```python
from build123d import *

# Parameters (mm, degrees)
DODANIE_WYCI_GNI_CIE1_DEPTH = 4
SZKIC2_R                    = 4
WYTNIJ_WYCI_GNI_CIE1_DEPTH  = 199.030300712


with BuildPart() as part:
    # Szkic1 → Dodanie-wyciągnięcie1 (new body)
    with BuildSketch(Plane(origin=(0, 0, 0), x_dir=(1, 0, 0), z_dir=(0, 1, 0))):
        with BuildLine():
            Line((-130, -140), (130, -140))
            ThreePointArc((130, -140), (137.071067812, -137.071067812), (140, -130))
            Line((140, -130), (140, 130))
            ThreePointArc((140, 130), (137.071067812, 137.071067812), (130, 140))
            Line((130, 140), (-130, 140))
            ThreePointArc((-130, 140), (-137.071067812, 137.071067812), (-140, 130))
            Line((-140, 130), (-140, -130))
            ThreePointArc((-140, -130), (-137.071067812, -137.071067812), (-130, -140))
        make_face()
    extrude(amount=DODANIE_WYCI_GNI_CIE1_DEPTH)

    # Szkic2 → Wytnij-wyciągnięcie1 (cut, through all)
    with BuildSketch(Plane(origin=(0, 4, 0), x_dir=(1, 0, 0), z_dir=(0, 1, 0))):
        with Locations(Location((120, 120, 0), (0, 0, 270))):
            Circle(SZKIC2_R)
        with Locations(Location((120, -120, 0), (0, 0, 270))):
            Circle(SZKIC2_R)
        with Locations(Location((-120, -120, 0), (0, 0, 270))):
            Circle(SZKIC2_R)
        with Locations(Location((-120, 120, 0), (0, 0, 270))):
            Circle(SZKIC2_R)
    extrude(amount=-WYTNIJ_WYCI_GNI_CIE1_DEPTH, mode=Mode.SUBTRACT)


solid = part.part
```
Work out the finished part from the listing and answer in its coordinate system (mm). Give positions to 0.01 mm unless a question says otherwise; leave off trailing zeros. Loops run counter-clockwise (first coordinate to the right, second up) from the corner with the lowest first, then second, coordinate; pieces in that order, holes last. Notation, with made-up numbers: (24, -37.75) - (35, -37.75) arc R15 cw to (35, -8.75) - close; hole circle Ø2 at (76, -1). An arc over 180 degrees is marked (long way). One line per question, with ' | ' between items.
(1) The mould has two halves that part along Z. Classify faces 1 (the face through (137.15, 1.97, -136.99)), 2 (the face through (-2, 4, -2)), 3 (the face through (123.373, 2.028, -117.85)): +Z half, -Z half, draft (parallel to the pull), parting line (faces both ways), or undercut.
Recorded:
face 1: -Z half | face 2: draft | face 3: undercut
(2) This flat-tipped pin is pushed along its axis until it touches: pin 1 Ø7 at (x, z) = (-120, -120) entering from -Y. Where does it stop, or does it pass through?
Recorded:
pin 1: passes through
(3) Straight lines are drawn through the part: probe 1 along X at (y, z) = (1.4, -120); probe 2 along Z at (x, y) = (122, 0.8). For each, find the intervals that lie inside material, in ascending order.
Recorded:
probe 1: x = -140 to -124, -116 to 116, 124 to 140 | probe 2: z = -140 to -123.46, -116.54 to 116.54, 123.46 to 140
(4) The part is cut by section B-B (x = -120). Write down the section's boundary in (y, z), then the cut area to 3 significant figures.
Recorded:
outline: (0, -140) - (4, -140) - (4, -124) - (0, -124) - close; (0, -116) - (4, -116) - (4, 116) - (0, 116) - close; (0, 124) - (4, 124) - (4, 140) - (0, 140) - close | area: 1,060 mm²
(5) The part is cut by section A-A (z = 120). Write down the section's boundary in (x, y), then the cut area to 3 significant figures.
Recorded:
outline: (-140, 0) - (-124, 0) - (-124, 4) - (-140, 4) - close; (-116, 0) - (116, 0) - (116, 4) - (-116, 4) - close; (124, 0) - (140, 0) - (140, 4) - (124, 4) - close | area: 1,060 mm²
